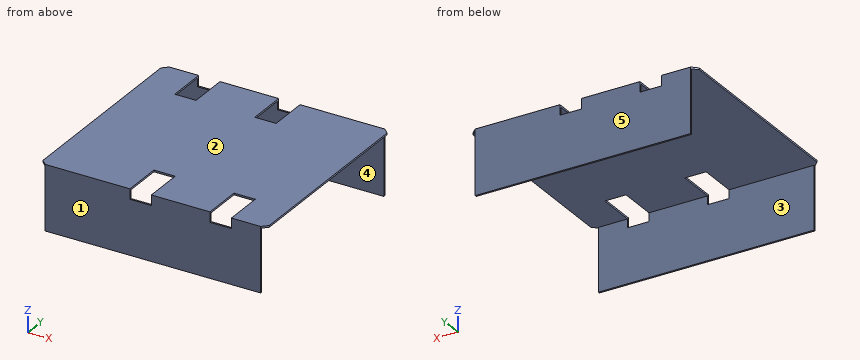
```python
from build123d import *

# Parameters (mm, degrees)
F_5052_START                               = 86
F_5052_SHEET_TOP_PANEL_DEPTH               = 1.6
FOLDED_START                               = 27
SKETCH2_W                                  = 202
SKETCH2_H                                  = 1.6
FOLDED_SIDE_SKIRTS_WITH_OPEN_ENDS_DEPTH    = 59
FOUR_START                                 = 78
SKETCH3_W                                  = 20
SKETCH3_H                                  = 38
FOUR_SIDE_OPEN_HOSE_AND_WRENCH_SLOTS_DEPTH = 9.6


with BuildPart() as part:
    # Sketch1 → 5052 sheet top panel (new body)
    with BuildSketch(Plane.XY.offset(F_5052_START)):
        Polygon((-101, -96), (101, -96), (106, -91), (106, 91), (101, 96), (-101, 96), (-106, 91), (-106, -91), align=None)
    extrude(amount=F_5052_SHEET_TOP_PANEL_DEPTH)

    # Sketch2 → Folded side skirts with open ends (add)
    with BuildSketch(Plane.XY.offset(FOLDED_START)):
        with Locations((0, 95.2)):
            Rectangle(SKETCH2_W, SKETCH2_H)
        with Locations((0, -95.2)):
            Rectangle(SKETCH2_W, SKETCH2_H)
    extrude(amount=FOLDED_SIDE_SKIRTS_WITH_OPEN_ENDS_DEPTH)

    # Sketch3 → Four side-open hose and wrench slots (cut)
    with BuildSketch(Plane.XY.offset(FOUR_START)):
        with Locations((-63.5, 78)):
            Rectangle(SKETCH3_W, SKETCH3_H)
        with Locations((63.5, -78)):
            Rectangle(SKETCH3_W, SKETCH3_H)
        with Locations((11.5, 78)):
            Rectangle(SKETCH3_W, SKETCH3_H)
        with Locations((-11.5, -78)):
            Rectangle(SKETCH3_W, SKETCH3_H)
    extrude(amount=FOUR_SIDE_OPEN_HOSE_AND_WRENCH_SLOTS_DEPTH, mode=Mode.SUBTRACT)


solid = part.part
```
Geometry check sheet. Reference: the model listing, model coordinates, mm. Face numbers are marked on the shaded views. A direction names the side the tool comes from. Coordinates: 2 decimals unless noted, no trailing zeros. Write each loop counter-clockwise with the first axis right and the second up, starting at its lowest first coordinate (ties: lowest second). Pieces come first, ordered by that corner, then holes. Notation, with made-up numbers: M 3.5,11.5 L 9.5,11.5 A27 cw 9.5,44.5 Z; hole C -12,24.25 d3. An arc over 180 degrees is marked long. Answer as a JSON object with one key per item and string values.
1. Tool access check on the marked faces 4 and 5. Record the directions out of +Z, -Z, +X, -X, +Y, -Y that give a thin tool (end or side, any length) a straight path to the whole face; none if there is none.
Answers below:
{"face 4": "-Z, +X, -X", "face 5": "+Z, -Z, +X, -X, +Y"}
2. Section check C-C, the plane x = 14.5. Enter the section's corners in (y, z).
Answers below:
{"outline": "M -96,27 L -94.4,27 L -94.4,86 L 59,86 L 59,87.6 L -96,87.6 Z; M 94.4,27 L 96,27 L 96,78 L 94.4,78 Z"}
3. Section check D-D, the plane x = -31.5. Enter the section's corners in (y, z).
Answers below:
{"outline": "M -96,27 L -94.4,27 L -94.4,86 L 94.4,86 L 94.4,27 L 96,27 L 96,87.6 L -96,87.6 Z"}
4. Section check B-B, the plane z = 39.5. Enter the section's corners in (x, y), plus the area to 3 significant figures.
Answers below:
{"outline": "M -101,-96 L 101,-96 L 101,-94.4 L -101,-94.4 Z; M -101,94.4 L 101,94.4 L 101,96 L -101,96 Z", "area": "646 mm²"}
5. Go/stop test with flat-tipped pins: pin 1 Ø0.5 at (y, z) = (-95, 60.5) entering from +X; pin 2 Ø0.5 at (x, y) = (-13, -95) entering from +Z; pin 3 Ø1.8 at (x, z) = (-14.5, 87) entering from -Y. Record where each tip stops, or that it passes through.
Answers below:
{"pin 1": "stops at x = 101", "pin 2": "stops at z = 78", "pin 3": "stops at y = -59"}
6. Scan lines: L1, parallel to Y at x = -75, z = 35; L2, parallel to Z at x = 57.5, y = 36; L3, parallel to Y at x = 59, z = 83.5. Record each from-to range of solid material in increasing order.
Answers below:
{"L1": "y = -96 to -94.4, 94.4 to 96", "L2": "z = 86 to 87.6", "L3": "y = 94.4 to 96"}
7. Draft check along Y on the marked faces 1, 2 and 3. Enter one of: released by +Y, released by -Y, zero draft, split by the parting line, or undercut.
Answers below:
{"face 1": "released by -Y", "face 2": "zero draft", "face 3": "undercut"}
8. Section check A-A, the plane y = -70.5. Enter the section's corners in (x, z), plus the area to 3 significant figures.
Answers below:
{"outline": "M -106,86 L -21.5,86 L -21.5,87.6 L -106,87.6 Z; M -1.5,86 L 53.5,86 L 53.5,87.6 L -1.5,87.6 Z; M 73.5,86 L 106,86 L 106,87.6 L 73.5,87.6 Z", "area": "275 mm²"}
